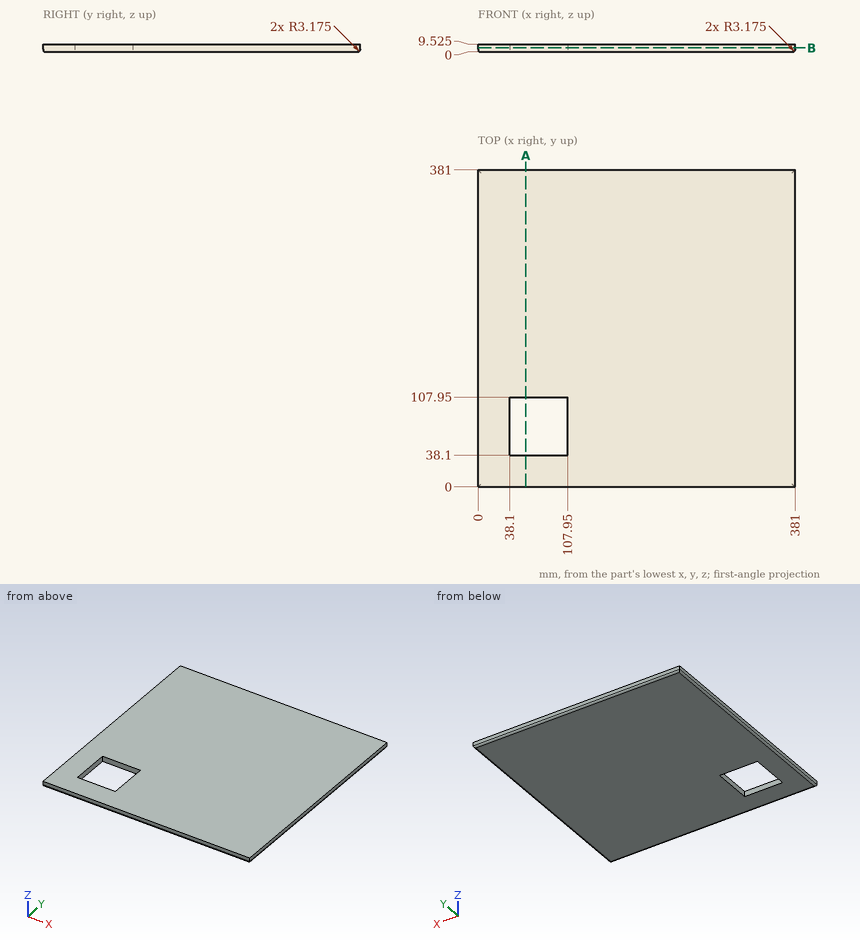
Answer from the drawing. Dimensions are ordinates in mm from the lowest x, y and z of the part. Give positions to 0.01 mm unless a question says otherwise; leave off trailing zeros. Loops run counter-clockwise (first coordinate to the right, second up) from the corner with the lowest first, then second, coordinate; pieces in that order, holes last. Notation, with made-up numbers: (10, 18.25) -> (66, 18.25) arc R16 ccw to (66, 40.25) -> close; hole circle Ø8 at (-13, 86). An arc over 180 degrees is marked (long way). Use a Markdown table: item, result.
Q1. Section A-A, the plane x = 57.5 is taken. Determine the outline of the cut face in (y, z) (3 decimals).
Solved:
| item | result |
|---|---|
| outline | (0, 3.175) arc R3.175 ccw to (3.175, 0) -> (38.1, 0) -> (38.1, 9.525) -> (0, 9.525) -> close; (107.95, 0) -> (377.825, 0) arc R3.175 ccw to (381, 3.175) -> (381, 9.525) -> (107.95, 9.525) -> close |
Q2. Each of these flat-tipped pins is pushed along its axis until it touches: pin 1 (1.5 mm diameter, centred on x = 63, y = 105.5, fed in from -Z); pin 2 (1 mm diameter, centred on x = 165.5, z = 2, fed in from -Y); pin 3 (1 mm diameter, centred on y = 236.5, z = 2.5, fed in from -X). Where does it stop, or does it pass through?
Solved:
| item | result |
|---|---|
| pin 1 | passes through |
| pin 2 | stops at y = 0.07 |
| pin 3 | stops at x = 0 |
Q3. Find the intervals of material crossed by line 1 along Y through (x, z) = (48.5, 7.75); line 2 along X through (y, z) = (293.5, 2.5), in increasing order.
Solved:
| item | result |
|---|---|
| line 1 | y = 0 to 38.1, 107.95 to 381 |
| line 2 | x = 0.07 to 380.93 |
Q4. Section B-B, the plane z = 4.75 is taken. Determine the outline of the cut face in (x, y), then the cut area to 3 significant figures.
Solved:
| item | result |
|---|---|
| outline | (0, 0) -> (381, 0) -> (381, 381) -> (0, 381) -> close; hole (38.1, 38.1) -> (107.95, 38.1) -> (107.95, 107.95) -> (38.1, 107.95) -> close |
| area | 140,000 mm^2 |
